Input: dimensioned drawing with shaded views. Units: mm. Origin: part minimum x, y, z. A direction names the side the tool comes from. Round coordinates to 2 decimals unless told otherwise and drop trailing zeros. Loops run counter-clockwise (first coordinate to the right, second up) from the corner with the lowest first, then second, coordinate; pieces in that order, holes last. Notation, with made-up numbers: M -21,87 L 0,87 A29 cw 0,118 Z; hole C 54,24 d3. An arc over 180 degrees is marked long. Put each result on its own line as item: value. Start each with the question number.
1) Section C-C on x = 9.5. Output: boundary loops of the cut face in (y, z).
2) Section A-A on z = 12.5. Output: boundary loops of the cut face in (x, y).
3) Pin query (flat end, axial travel): pin 1 (3 mm diameter, centred on x = 7.5, y = 4.5, fed in from -Z); pin 2 (1 mm diameter, centred on x = 9.5, y = 16.5, fed in from -Z); pin 3 (4 mm diameter, centred on x = 6, z = 10, fed in from +Y). Return the tip coordinate at first contact, or that it passes through.
4) Section D-D on z = 7.25. Output: boundary loops of the cut face in (x, y).
5) Section B-B on y = 16.5. Output: boundary loops of the cut face in (x, z), plus the area to 3 significant figures.
6) Reachability of the marked faces 1 and 2 from +Z, -Z, +X, -X, +Y, -Y: full face, straight path, thin tool, end or side. Return the list, or none.
7) Draft query along Z for the marked faces 3, 4 and 5. Return one class per face: +Z half, -Z half, draft (parallel to the pull), parting line (faces both ways), or undercut.
8) Line query: probe 1 along Y at (x, z) = (11.25, 12.5); probe 2 along Y at (x, z) = (6.5, 12.75); probe 3 along X at (y, z) = (8.5, 3). Output: solid intervals per line, ascending.
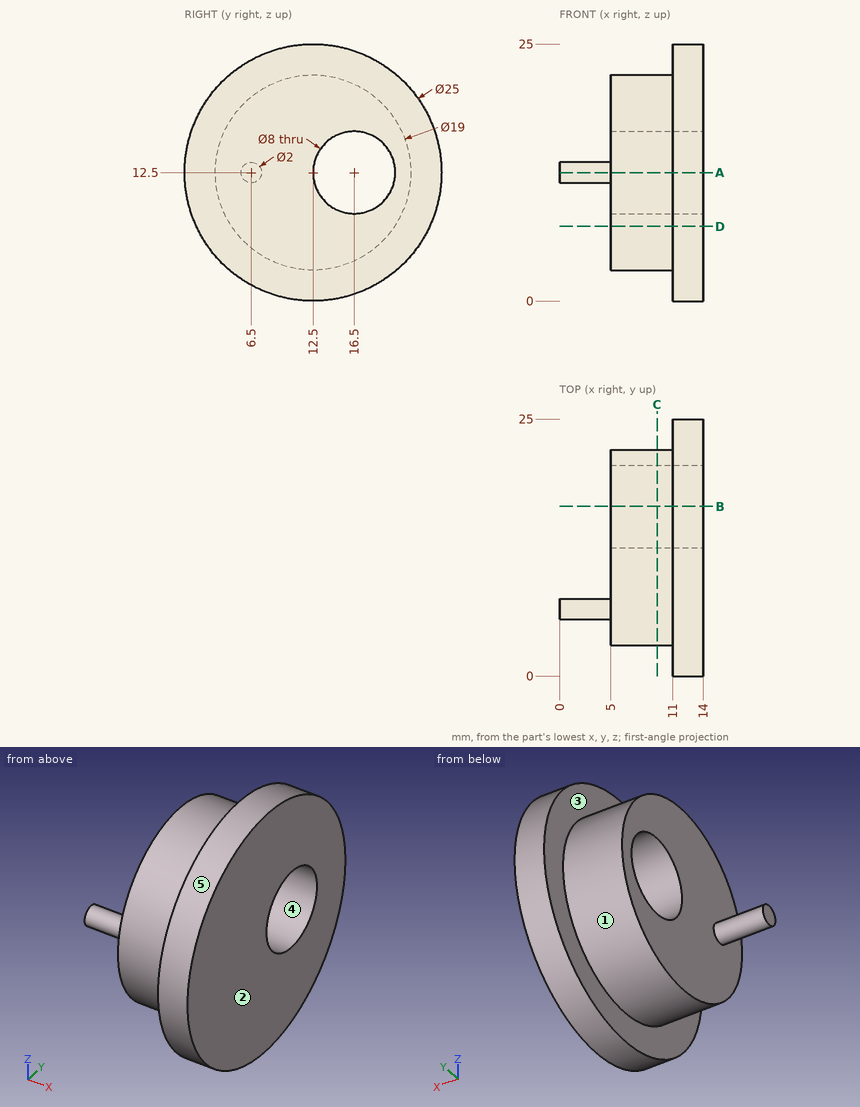
Geometry results:
1. outline: C 12.5,12.5 d19; hole C 16.5,12.5 d8
2. outline: M 0,5.5 L 5,5.5 L 5,3 L 11,3 L 11,0 L 14,0 L 14,12.5 L 5,12.5 L 5,7.5 L 0,7.5 Z; M 5,20.5 L 14,20.5 L 14,25 L 11,25 L 11,22 L 5,22 Z
3. pin 1: stops at z = 5.57
3. pin 2: stops at z = 3.67
3. pin 3: stops at y = 21.99
4. outline: M 5,4.58 L 11,4.58 L 11,1.16 L 14,1.16 L 14,23.84 L 11,23.84 L 11,20.42 L 5,20.42 Z
5. outline: M 5,3.88 L 11,3.88 L 11,0.66 L 14,0.66 L 14,8.5 L 5,8.5 Z; M 5,16.5 L 14,16.5 L 14,24.34 L 11,24.34 L 11,21.12 L 5,21.12 Z
5. area: 102 mm²
6. face 1: -X
6. face 2: +Z, -Z, +X, +Y, -Y
7. face 3: draft
7. face 4: undercut
7. face 5: parting line
8. probe 1: y = 0 to 12.5, 20.5 to 25
8. probe 2: y = 3 to 12.51, 20.49 to 22
8. probe 3: x = 11 to 14
